```python
from build123d import *

# Parameters (mm, degrees)
BOSS_EXTRUDE1_DEPTH = 15
SKETCH2_R           = 4
CUT_EXTRUDE1_DEPTH  = 160.628474903


with BuildPart() as part:
    # Sketch1 → Boss-Extrude1 (new, symmetric)
    with BuildSketch(Plane(origin=(0, 0, 0), x_dir=(1, 0, 0), z_dir=(0, 1, 0))):
        Polygon((50.5, -2), (50.5, -150), (52.5, -150), (52.5, 0), (-52.5, 0), (-52.5, -150), (-50.5, -150), (-50.5, -2), align=None)
    extrude(amount=BOSS_EXTRUDE1_DEPTH, both=True)

    # Sketch2 → Cut-Extrude1 (cut, through all)
    with BuildSketch(Plane(origin=(0, 0, 0), x_dir=(-1, 0, 0), z_dir=(0, 0, -1))):
        Circle(SKETCH2_R)
    extrude(amount=-CUT_EXTRUDE1_DEPTH, mode=Mode.SUBTRACT)


solid = part.part
```
Design review of the part built by this model. Coordinates are the model's own, in mm. A direction names the side the tool comes from. Round coordinates to 2 decimals unless told otherwise and drop trailing zeros. Order: outer loops, then holes, each group sorted by start corner. A loop starts at its lowest first (then second) coordinate and runs counter-clockwise, first axis right, second up. Notation, with made-up numbers: (7.5, -37.75) - (26.5, -37.75) arc R15 ccw to (26.5, -12.75) - close; hole circle Ø4 at (23, -26.5). An arc over 180 degrees is marked (long way). Return JSON: item names as keys, results as strings.
Q1. Consider section A-A on x = 0. Write out the cut boundary in (y, z).
Computed values:
{"outline": "(-15, 0) - (-4, 0) - (-4, 2) - (-15, 2) - close; (4, 0) - (15, 0) - (15, 2) - (4, 2) - close"}
Q2. For pin 1 Ø13 at (x, y) = (0, 0) entering from -Z; pin 2 Ø12 at (x, y) = (33.5, 2) entering from +Z, all flat-tipped, find the tip position at first contact; note any pin that passes through.
Computed values:
{"pin 1": "stops at z = 0", "pin 2": "stops at z = 2"}
Q3. Consider section B-B on y = 0. Write out the cut boundary in (x, z), plus the area to 3 significant figures.
Computed values:
{"outline": "(-52.5, 0) - (-4, 0) - (-4, 2) - (-50.5, 2) - (-50.5, 150) - (-52.5, 150) - close; (4, 0) - (52.5, 0) - (52.5, 150) - (50.5, 150) - (50.5, 2) - (4, 2) - close", "area": "786 mm2"}
Q4. The part is to be moulded in two halves that separate along Y. For faces 1 (the cylindrical face through (0.867, -3.905, 0.986)), 2 (the flat face through (-51, -15, 75)), 3 (the flat face through (1, 7, 0)), say which applies: pulls with the +Y half, pulls with the -Y half, needs draft (parallel to the pull), parting line crosses it, or undercut.
Computed values:
{"face 1": "undercut", "face 2": "pulls with the -Y half", "face 3": "needs draft"}
Q5. Machinability: for faces 4 (the flat face through (-1, 7, 2)), 5 (the flat face through (-51, 15, 75)), which of the approach directions +Z, -Z, +X, -X, +Y, -Y give a long, thin tool a straight path to every point of the face, cutting with its end or side? Answer none if there is none.
Computed values:
{"face 4": "+Z, +Y, -Y", "face 5": "+Z, -Z, +X, -X, +Y"}
Q6. Consider section D-D on y = 7.25. Write out the cut boundary in (x, z), plus the area to 3 significant figures.
Computed values:
{"outline": "(-52.5, 0) - (52.5, 0) - (52.5, 150) - (50.5, 150) - (50.5, 2) - (-50.5, 2) - (-50.5, 150) - (-52.5, 150) - close", "area": "802 mm2"}
Q7. Wall thickness on L1, parallel to X at y = 11.5, z = 108; L2, parallel to Y at x = 0, z = 1.55; L3, parallel to Z at x = -47, y = -5.5: over which ranges is each line inside the solid? List them lowest first. Write a range as [from, to].
Computed values:
{"L1": "x = [-52.5, -50.5], [50.5, 52.5]", "L2": "y = [-15, -4], [4, 15]", "L3": "z = [0, 2]"}
Q8. Consider section C-C on z = 123.5. Write out the cut boundary in (x, y), plus the area to 3 significant figures.
Computed values:
{"outline": "(-52.5, -15) - (-50.5, -15) - (-50.5, 15) - (-52.5, 15) - close; (50.5, -15) - (52.5, -15) - (52.5, 15) - (50.5, 15) - close", "area": "120 mm2"}
